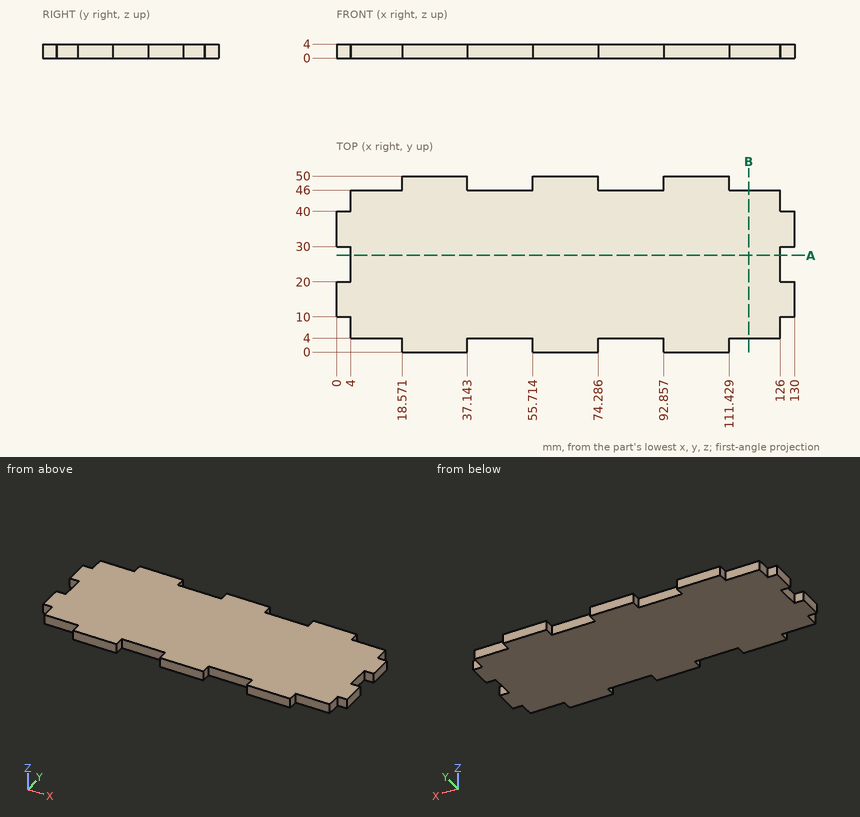
Job drawing, mm, ordinate dimensions from the low corner. One solid piece. Round coordinates to 2 decimals unless told otherwise and drop trailing zeros. Loops run counter-clockwise (first coordinate to the right, second up) from the corner with the lowest first, then second, coordinate; pieces in that order, holes last.
(1) Wall check: line 1 along X through (y, z) = (47.5, 1.45) (1 decimal); line 2 along X through (y, z) = (42, 1.05); line 3 along Y through (x, z) = (53.5, 3.65). Give the ranges that are in metal, low to high.
(2) Cut at B-B (x = 117). Give the cut face in (y, z), plus the area to 3 significant figures.
(3) Cut at A-A (y = 27.5). Give the cut face in (x, z), plus the area to 3 significant figures.
(4) Drop flat-ended pins along their axis: pin 1 (1.2 mm diameter, centred on x = 128.5, z = 2, fed in from -Y); pin 2 (4 mm diameter, centred on x = 76, y = 22, fed in from -Z); pin 3 (1.2 mm diameter, centred on y = 26, z = 1, fed in from +X); pin 4 (1.2 mm diameter, centred on y = 48.5, z = 1.5, fed in from +X). Give the stop position or say it passes through.
Findings below:
1. line 1: x = 18.6 to 37.1, 55.7 to 74.3, 92.9 to 111.4
1. line 2: x = 4 to 126
1. line 3: y = 4 to 46
2. outline: (4, 0) - (46, 0) - (46, 4) - (4, 4) - close
2. area: 168 mm2
3. outline: (4, 0) - (126, 0) - (126, 4) - (4, 4) - close
3. area: 488 mm2
4. pin 1: stops at y = 10
4. pin 2: stops at z = 0
4. pin 3: stops at x = 126
4. pin 4: stops at x = 111.43
